Answer from the drawing. Dimensions are ordinates in mm from the lowest x, y and z of the part. A direction names the side the tool comes from. Coordinates: 2 decimals unless noted, no trailing zeros. Loops run counter-clockwise (first coordinate to the right, second up) from the corner with the lowest first, then second, coordinate; pieces in that order, holes last.
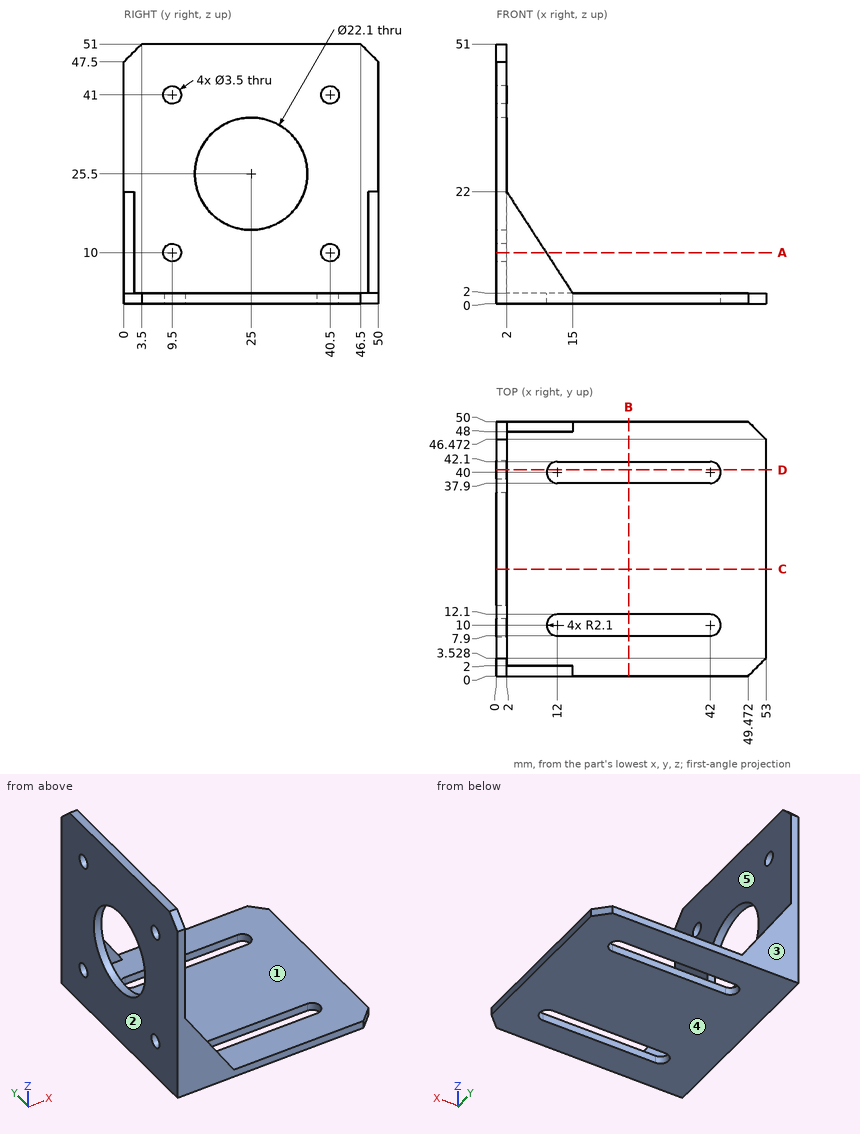
Item 1: A cutting plane is placed at C-C on y = 21. Determine the outline of the cut face in (x, z).
Numbers:
outline: (0, 0) - (53, 0) - (53, 2) - (2, 2) - (2, 15.2) - (0, 15.2) - close; (0, 35.8) - (2, 35.8) - (2, 51) - (0, 51) - close
Item 2: Find the intervals of material crossed by line 1 along Z through (x, y) = (0.85, 40.5); line 2 along Y through (x, z) = (1.25, 25.5); line 3 along Z through (x, y) = (27, 33), in increasing order.
Numbers:
line 1: z = 0 to 8.25, 11.75 to 39.25, 42.75 to 51
line 2: y = 0 to 13.95, 36.05 to 50
line 3: z = 0 to 2
Item 3: Determine the mould class of the marked faces 1, 2 and 3 for opening direction Y: released by +Y, released by -Y, zero draft, split by the parting line, or undercut.
Numbers:
face 1: undercut
face 2: zero draft
face 3: released by +Y
Item 4: Given pin 1 (4 mm diameter, centred on x = 9.5, z = 16.5, fed in from +Y); pin 2 (12 mm diameter, centred on y = 36, z = 38.5, fed in from +X); pin 3 (1 mm diameter, centred on x = 16.5, y = 35, fed in from +Z), each flat-ended and moving along its own axis, determine where each tip first touches the part or whether it passes through.
Numbers:
pin 1: passes through
pin 2: stops at x = 2
pin 3: stops at z = 2
Item 5: A cutting plane is placed at A-A on z = 10. Determine the outline of the cut face in (x, y), then the cut area to 3 significant figures.
Numbers:
outline: (0, 0) - (9.8, 0) - (9.8, 2) - (2, 2) - (2, 7.75) - (0, 7.75) - close; (0, 11.25) - (2, 11.25) - (2, 38.75) - (0, 38.75) - close; (0, 42.25) - (2, 42.25) - (2, 48) - (9.8, 48) - (9.8, 50) - (0, 50) - close
area: 117 mm2
Item 6: Which of the six approach directions +Z, -Z, +X, -X, +Y, -Y give full straight-line access (tool end or side, diameter ignored) to the marked faces 4 and 5?
Numbers:
face 4: -Z, +X, -X, +Y, -Y
face 5: +Z, +X
Item 7: A cutting plane is placed at B-B on x = 26. Determine the outline of the cut face in (y, z).
Numbers:
outline: (0, 0) - (7.9, 0) - (7.9, 2) - (0, 2) - close; (12.1, 0) - (37.9, 0) - (37.9, 2) - (12.1, 2) - close; (42.1, 0) - (50, 0) - (50, 2) - (42.1, 2) - close
Item 8: A cutting plane is placed at D-D on y = 40.5. Determine the outline of the cut face in (x, z), then the cut area to 3 significant figures.
Numbers:
outline: (0, 0) - (9.96, 0) - (9.96, 2) - (2, 2) - (2, 8.25) - (0, 8.25) - close; (0, 11.75) - (2, 11.75) - (2, 39.25) - (0, 39.25) - close; (0, 42.75) - (2, 42.75) - (2, 51) - (0, 51) - close; (44.04, 0) - (53, 0) - (53, 2) - (44.04, 2) - close
area: 122 mm2
